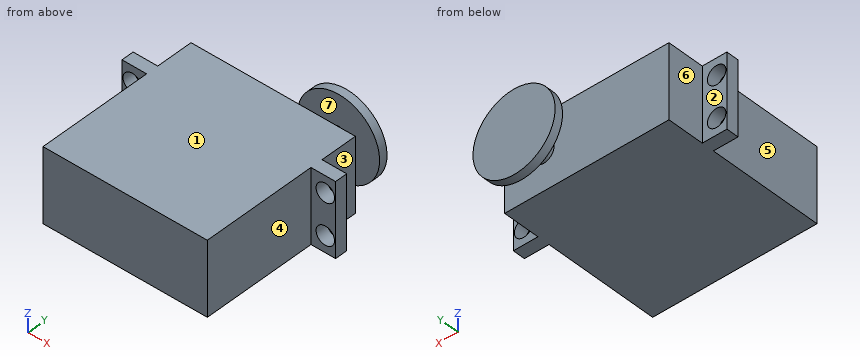
```python
from build123d import *

# Parameters (mm, degrees)
SKETCH1_W           = 40
SKETCH1_H           = 18
BOSS_EXTRUDE1_DEPTH = 40
SKETCH2_W           = 6
SKETCH2_H           = 18
BOSS_EXTRUDE2_DEPTH = 3
SKETCH3_R           = 2.5
BOSS_EXTRUDE3_DEPTH = 6
SKETCH4_R           = 10
BOSS_EXTRUDE4_DEPTH = 2
CUT_EXTRUDE1_REACH  = 60.634
SKETCH5_R           = 2.25


with BuildPart() as part:
    # Sketch1 → Boss-Extrude1 (new body)
    with BuildSketch(Plane(origin=(0, 0, 0), x_dir=(1, 0, 0), z_dir=(0, 1, 0))):
        with Locations((20, 9)):
            Rectangle(SKETCH1_W, SKETCH1_H)
    extrude(amount=BOSS_EXTRUDE1_DEPTH)

    # Sketch2 → Boss-Extrude2 (add)
    with BuildSketch(Plane(origin=(0, 28, 0), x_dir=(-1, 0, 0), z_dir=(0, -1, 0))):
        with Locations((3, 9)):
            Rectangle(SKETCH2_W, SKETCH2_H)
        with Locations((-43, 9)):
            Rectangle(SKETCH2_W, SKETCH2_H)
    extrude(amount=-BOSS_EXTRUDE2_DEPTH)

    # Sketch3 → Boss-Extrude3 (add)
    with BuildSketch(Plane(origin=(0, 40, 0), x_dir=(1, 0, 0), z_dir=(0, 1, 0))):
        with Locations(Location((30.5, 9, 0), (0, 0, 90))):
            Circle(SKETCH3_R)
    extrude(amount=BOSS_EXTRUDE3_DEPTH)

    # Sketch4 → Boss-Extrude4 (add)
    with BuildSketch(Plane(origin=(0, 46, 0), x_dir=(1, 0, 0), z_dir=(0, 1, 0))):
        with Locations(Location((30.5, 9, 0), (0, 0, 270))):
            Circle(SKETCH4_R)
    extrude(amount=BOSS_EXTRUDE4_DEPTH)

    # Sketch5 → Cut-Extrude1 (cut, up to next)
    with BuildSketch(Plane(origin=(0, 31, 0), x_dir=(1, 0, 0), z_dir=(0, 1, 0)), mode=Mode.PRIVATE) as cut_extrude1_sk1:
        with Locations(Location((-3.5, 14, 0), (0, 0, 270))):
            Circle(SKETCH5_R)
    cut_extrude1_tool1 = extrude(cut_extrude1_sk1.sketch, amount=-CUT_EXTRUDE1_REACH, mode=Mode.PRIVATE) & part.part
    # Sketch5 → Cut-Extrude1 (cut, up to next)
    with BuildSketch(Plane(origin=(0, 31, 0), x_dir=(1, 0, 0), z_dir=(0, 1, 0)), mode=Mode.PRIVATE) as cut_extrude1_sk2:
        with Locations(Location((-3.5, 4, 0), (0, 0, 270))):
            Circle(SKETCH5_R)
    cut_extrude1_tool2 = extrude(cut_extrude1_sk2.sketch, amount=-CUT_EXTRUDE1_REACH, mode=Mode.PRIVATE) & part.part
    cut_extrude1_1 = cut_extrude1_tool1.solids().sort_by_distance((-3.5, 31, -14))[0]
    add(cut_extrude1_1, mode=Mode.SUBTRACT)
    cut_extrude1_2 = cut_extrude1_tool2.solids().sort_by_distance((-3.5, 31, -4))[0]
    add(cut_extrude1_2, mode=Mode.SUBTRACT)
    cut_extrude1 = cut_extrude1_1 + cut_extrude1_2  # Cut-Extrude1 as one shape, for the pattern or mirror that repeats it

    # Mirror1: Cut-Extrude1 across plane
    add(cut_extrude1.mirror(Plane.ZY.offset(-20)), mode=Mode.SUBTRACT)


solid = part.part
```
Source: CAD feature listing. Evaluate the final solid. Frame: model axes, mm. Face numbers are marked on the shaded views. A direction names the side the tool comes from. Coordinates: 2 decimals unless noted, no trailing zeros. Write each loop counter-clockwise with the first axis right and the second up, starting at its lowest first coordinate (ties: lowest second). Pieces come first, ordered by that corner, then holes. Notation, with made-up numbers: (-6, 59.5) - (46, 59.5) arc R4 cw to (46, 64.5) - close; hole circle Ø1 at (-4, 48). An arc over 180 degrees is marked (long way). Answer as a JSON object with one key per item and string values.
Q1. Section query C-C, the plane x = 30.5. Output: boundary loops of the cut face in (y, z), plus the area to 3 significant figures.
Ans:
{"outline": "(0, -18) - (40, -18) - (40, -11.5) - (46, -11.5) - (46, -19) - (48, -19) - (48, 1) - (46, 1) - (46, -6.5) - (40, -6.5) - (40, 0) - (0, 0) - close", "area": "790 mm2"}
Q2. Section query D-D, the plane z = -9. Output: boundary loops of the cut face in (x, y).
Ans:
{"outline": "(-6, 28) - (0, 28) - (0, 0) - (40, 0) - (40, 28) - (46, 28) - (46, 31) - (40, 31) - (40, 40) - (33, 40) - (33, 46) - (40.5, 46) - (40.5, 48) - (20.5, 48) - (20.5, 46) - (28, 46) - (28, 40) - (0, 40) - (0, 31) - (-6, 31) - close"}
Q3. Set-up query: the marked faces 4, 5, 6 and 7. Return all of +Z, -Z, +X, -X, +Y, -Y with unobstructed straight access to the full face (end or side cutting, diameter ignored); none if empty.
Ans:
{"face 4": "+Z, -Z, +X, -Y", "face 5": "+Z, -Z, -X, -Y", "face 6": "+Z, -Z, -X, +Y", "face 7": "none"}
Q4. Section query B-B, the plane z = -5. Output: boundary loops of the cut face in (x, y), plus the area to 3 significant figures.
Ans:
{"outline": "(-6, 28) - (-5.52, 28) - (-5.52, 31) - (-6, 31) - close; (-1.48, 28) - (0, 28) - (0, 0) - (40, 0) - (40, 28) - (41.48, 28) - (41.48, 31) - (40, 31) - (40, 40) - (0, 40) - (0, 31) - (-1.48, 31) - close; (21.33, 46) - (39.67, 46) - (39.67, 48) - (21.33, 48) - close; (45.52, 28) - (46, 28) - (46, 31) - (45.52, 31) - close", "area": "1,650 mm2"}
Q5. Material intervals for line 1 (X direction, y = 28.8, z = -14); line 2 (Y direction, x = 23.5, z = -7.5); line 3 (X direction, y = 14.5, z = -10.5), sorted ascending. Write a range as [from, to].
Ans:
{"line 1": "x = [-6, -5.75], [-1.25, 41.25], [45.75, 46]", "line 2": "y = [0, 40], [46, 48]", "line 3": "x = [0, 40]"}
Q6. First-contact query: pin 1 Ø5 at (x, y) = (5.5, 11.5) entering from +Z; pin 2 Ø4 at (y, z) = (15.5, -3.5) entering from +X; pin 3 Ø12 at (x, z) = (-0.5, -9) entering from +Y. Flat tips, straight axial feed; report the tip coordinate or a pass-through.
Ans:
{"pin 1": "stops at z = 0", "pin 2": "stops at x = 40", "pin 3": "stops at y = 40"}
Q7. Section query A-A, the plane x = 43.5. Output: boundary loops of the cut face in (y, z).
Ans:
{"outline": "(28, -18) - (31, -18) - (31, -16.25) - (28, -16.25) - close; (28, -11.75) - (31, -11.75) - (31, -6.25) - (28, -6.25) - close; (28, -1.75) - (31, -1.75) - (31, 0) - (28, 0) - close"}
Q8. Draft query along Y for the marked faces 1, 2 and 3. Return one class per face: released by +Y, released by -Y, zero draft, split by the parting line, or undercut.
Ans:
{"face 1": "zero draft", "face 2": "released by +Y", "face 3": "undercut"}
